Read the model definition and answer for the solid it produces. Units are mm, in the model's axes. A direction names the side the tool comes from. Coordinates: 2 decimals unless noted, no trailing zeros. Write each loop counter-clockwise with the first axis right and the second up, starting at its lowest first coordinate (ties: lowest second). Pieces come first, ordered by that corner, then holes.
1) Each of these flat-tipped pins is pushed along its axis until it touches: pin 1 Ø8 at (x, z) = (-0.5, 7.5) entering from +Y; pin 2 Ø12 at (y, z) = (-24, -1) entering from -X; pin 3 Ø4 at (x, y) = (4, -16) entering from +Z; pin 4 Ø10 at (y, z) = (-27.5, -6) entering from +X. Where does it stop, or does it pass through?
2) Find the intervals of material crossed by line 1 (Y direction, x = 1.5, z = 19); line 2 (Z direction, x = -2, y = -16.5); line 3 (Z direction, x = 7.5, y = -9), in increasing order.
3) The part is cut by section C-C (y = -12). Determine the outline of the cut face in (x, z).
4) Which of the six approach directions +Z, -Z, +X, -X, +Y, -Y give full straight-line access (tool end or side, diameter ignored) to faces 1 (the face through (4.02, -22.68, 1.27)), 2 (the face through (0, 0, 0))?
from build123d import *

# Parameters (mm, degrees)
F0_R     = 25.4
F1_DEPTH = 10.16
F2_R     = 5.08
F3_R     = 5.07999
F4_R     = 4.2168312207
F5_DEPTH = 25.4


# Not quite as in the source:
# - a fillet or chamfer is up to 0.001 mm smaller than in the source, because OpenCascade refuses the exact size


with BuildPart() as f1:
    # F0 (on Front) → F1 (new body)
    with BuildSketch(Plane.XZ):
        Circle(F0_R)
    extrude(amount=F1_DEPTH)

    # F2
    f2_edges = [f1.edges().sort_by_distance(p)[0] for p in [
        (-25.4, -10.16, 0),
    ]]
    fillet(f2_edges, radius=F2_R)

    # F3 (radius 5.08 in the source; OpenCascade refuses exactly that, so slightly less here)
    f3_edges = [f1.edges().sort_by_distance(p)[0] for p in [
        (-25.4, 0, 0),
    ]]
    fillet(f3_edges, radius=F3_R)

    # F4 (on face) → F5 (join)
    with BuildSketch(Plane.XZ.offset(10.16)):
        Circle(F4_R)
    extrude(amount=F5_DEPTH)


solid = f1.part
Reported:
1. pin 1: stops at y = 0
1. pin 2: stops at x = -4.22
1. pin 3: stops at z = 3.71
1. pin 4: stops at x = 4.1
2. line 1: y = -10.16 to 0
2. line 2: z = -3.71 to 3.71
2. line 3: z = -22.32 to 22.32
3. outline: circle Ø8.43 at (0, 0)
4. face 1: -Y
4. face 2: +Z, -Z, +X, -X, +Y
